Geometry check sheet. Reference: the model listing, model coordinates, mm. A direction names the side the tool comes from. Round coordinates to 2 decimals unless told otherwise and drop trailing zeros. Order: outer loops, then holes, each group sorted by start corner. A loop starts at its lowest first (then second) coordinate and runs counter-clockwise, first axis right, second up.
(1) Set-up check for faces 1 (the face through (-75.98, -24.65, 1.67)), 2 (the face through (127, -7, -10)): record each of +Z, -Z, +X, -X, +Y, -Y from which the full face is reachable in a straight line by a thin tool's end or side.
(2) Cross-section at A-A on z = 0. Enter the section's corners in (x, y), and give its area (3 significant figures).
(3) Cross-section at D-D on z = -33. Enter the section's corners in (x, y), and give its area (3 significant figures).
(4) Cross-section at B-B on y = -46. Enter the section's corners in (x, z), and give its area (3 significant figures).
(5) Draft check along Y on faces 3 (the face through (54, 0, 1)), 4 (the face through (-20.633, -11.605, -15.821)), 5 (the face through (55, -50, -67)). Enter one of: pulls with the +Y half, pulls with the -Y half, needs draft (parallel to the pull), parting line crosses it, or undercut.
(6) Thickness scan on L1, parallel to Z at x = 11.5, y = -31; L2, parallel to X at y = -3.1, z = 0; L3, parallel to Y at x = -50.5, z = -33. Record the ranges inside material, lowest first.
(7) Gauge pin test, flat ends, axial feed: P1, Ø12, axis at y = -22, z = 32, coming from the +X side; P2, Ø1.5, axis at y = -21.5, z = 50, coming from the +X side; P3, Ø4, axis at x = -28, z = 19.5, coming from the -Y side. Record the tip position at first contact, or that the pin passes through.
(8) Cross-section at C-C on y = -9.5. Enter the section's corners in (x, z), and give its area (3 significant figures).
from build123d import *

# Parameters (mm, degrees)
F2_DEPTH = 50
F4_DEPTH = 31
F5_R     = 26
F6_DEPTH = 15
F9_ANGLE = -360


with BuildPart() as f2:
    # F0 (on Front) → F2 (new body)
    with BuildSketch(Plane.XZ):
        with BuildLine():
            Line((111, 76), (0, 76))
            ThreePointArc((0, 76), (-76, 0), (0, -76))
            Line((0, -76), (111, -76))
            ThreePointArc((111, -76), (187, 0), (111, 76))
        make_face()
    extrude(amount=F2_DEPTH)

    # F3 (on offset) → F4 (cut)
    with BuildSketch(Plane.XZ.offset(19)):
        with BuildLine():
            Line((111, 64), (0, 64))
            ThreePointArc((0, 64), (-64, 0), (0, -64))
            Line((0, -64), (111, -64))
            ThreePointArc((111, -64), (175, 0), (111, 64))
        make_face()
    extrude(amount=F4_DEPTH, mode=Mode.SUBTRACT)

    # F5 (on offset) → F6 (cut)
    with BuildSketch(Plane.XZ.offset(19)):
        Circle(F5_R)
    extrude(amount=-F6_DEPTH, mode=Mode.SUBTRACT)

    # F8 (on offset) → F9 (revolve, symmetric, cut)
    with BuildSketch(Plane.YZ.offset(111)) as f9_sk:
        Polygon((-19, 0), (0, 0), (0, 11), (-2, 11), (-2, 18.5), (-7, 18.5), (-7, 23.5), (-19, 23.5), align=None)
    revolve(axis=Axis((111, -9.5, 0), (0, -1, 0)), revolution_arc=F9_ANGLE / 2, mode=Mode.SUBTRACT)
    revolve(f9_sk.sketch, axis=Axis((111, -9.5, 0), (0, 1, 0)), revolution_arc=F9_ANGLE / 2, mode=Mode.SUBTRACT)


solid = f2.part
Found:
1. face 1: -X, +Y, -Y
1. face 2: -Y
2. outline: (-76, -50) - (-64, -50) - (-64, -19) - (-26, -19) - (-26, -4) - (26, -4) - (26, -19) - (87.5, -19) - (87.5, -7) - (92.5, -7) - (92.5, -2) - (100, -2) - (100, 0) - (-76, 0) - close; (122, -2) - (129.5, -2) - (129.5, -7) - (134.5, -7) - (134.5, -19) - (175, -19) - (175, -50) - (187, -50) - (187, 0) - (122, 0) - close
2. area: 4,170 mm2
3. outline: (-68.46, -50) - (-54.84, -50) - (-54.84, -19) - (165.84, -19) - (165.84, -50) - (179.46, -50) - (179.46, 0) - (-68.46, 0) - close
3. area: 5,560 mm2
4. outline: (0, -76) - (111, -76) arc R76 ccw to (111, 76) - (0, 76) arc R76 ccw to start; hole (0, -64) - (111, -64) arc R64 ccw to (111, 64) - (0, 64) arc R64 ccw to start
4. area: 7,940 mm2
5. face 3: pulls with the +Y half
5. face 4: needs draft
5. face 5: pulls with the -Y half
6. L1: z = -76 to -64, 64 to 76
6. L2: x = -76 to 92.5, 129.5 to 187
6. L3: y = -19 to 0
7. P1: stops at x = 182.41
7. P2: stops at x = 168.88
7. P3: stops at y = -19
8. outline: (0, -76) - (111, -76) arc R76 ccw to (111, 76) - (0, 76) arc R76 ccw to start; hole circle Ø52 at (0, 0); hole circle Ø47 at (111, 0)
8. area: 31,200 mm2
